Read the model definition and answer for the solid it produces. Units are mm, in the model's axes. Face numbers are marked on the shaded views. A direction names the side the tool comes from. Round coordinates to 2 decimals unless told otherwise and drop trailing zeros. Write each loop counter-clockwise with the first axis right and the second up, starting at its lowest first coordinate (ties: lowest second). Pieces come first, ordered by that corner, then holes. Notation, with made-up numbers: (-9.75, 64) - (19.25, 64) arc R13 ccw to (19.25, 72) - close; hole circle Ø7 at (20.25, 33). An arc over 180 degrees is marked (long way). Answer as CSV lines item,"result". Start each with the question number.
1) Find section B-B on y = 3. Determine the outline of the cut face in (x, z), then the cut area to 3 significant figures.
2) Which of the six approach directions +Z, -Z, +X, -X, +Y, -Y give full straight-line access (tool end or side, diameter ignored) to the marked faces 1, 2 and 3?
3) Find section D-D on x = 53.5. Determine the outline of the cut face in (y, z), then the cut area to 3 significant figures.
4) Each of these flat-tipped pins is pushed along its axis until it touches: pin 1 (6 mm diameter, centred on y = 9.5, z = 21.5, fed in from +X); pin 2 (16 mm diameter, centred on y = 26.5, z = 20, fed in from -X); pin 3 (4 mm diameter, centred on x = 53.5, y = 14.5, fed in from +Z). Where does it stop, or does it pass through?
5) Find section C-C on z = 18. Determine the outline of the cut face in (x, y), then the cut area to 3 significant figures.
6) Find section A-A on x = 2.8. Determine the outline of the cut face in (y, z).
7) Consider line 1 along Y through (x, z) = (53.5, 2.9); line 2 along Y through (x, z) = (2.8, 3.4); line 3 along Y through (x, z) = (48.5, 31.5). Determine where each line is inside the solid, lowest interval first.
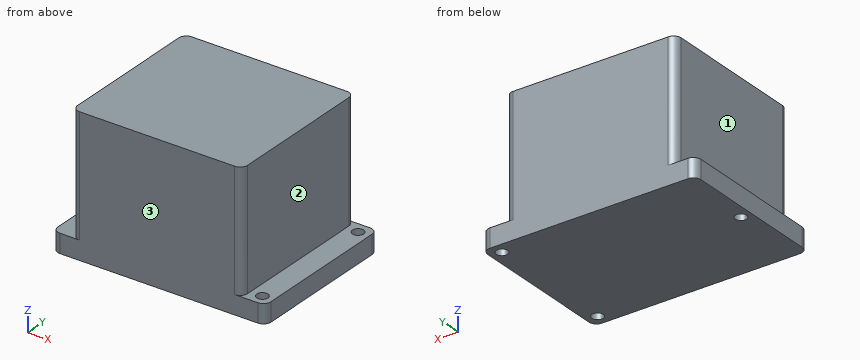
from build123d import *

# Parameters (mm, degrees)
SKETCH_1_W      = 56.5
SKETCH_1_H      = 41
SKETCH_1_R      = 1.5
EXTRUDE_1_DEPTH = 5
FILLET_1_R      = 2
SKETCH_2_W      = 45.103373127
SKETCH_2_H      = 41
EXTRUDE_2_DEPTH = 31.5
FILLET_2_R      = 2


with BuildPart() as part:
    # 草图1 → 凸台-拉伸1 (new body)
    with BuildSketch(Plane.XY):
        with Locations((28.25, 20.5)):
            Rectangle(SKETCH_1_W, SKETCH_1_H)
        with Locations((2.8, 20.5)):
            Circle(SKETCH_1_R, mode=Mode.SUBTRACT)
        with Locations((53.5, 38)):
            Circle(SKETCH_1_R, mode=Mode.SUBTRACT)
        with Locations((53.5, 3)):
            Circle(SKETCH_1_R, mode=Mode.SUBTRACT)
    extrude(amount=EXTRUDE_1_DEPTH)

    # 圆角1
    fillet_1_edges = [part.edges().sort_by_distance(p)[0] for p in [
        (0, 41, 2.5),
        (56.5, 41, 2.5),
        (56.5, 0, 2.5),
        (0, 0, 2.5),
    ]]
    fillet(fillet_1_edges, radius=FILLET_1_R)

    # 草图2 → 凸台-拉伸2 (add)
    with BuildSketch(Plane.XY.offset(5)):
        with Locations((27.783569507, 20.5)):
            Rectangle(SKETCH_2_W, SKETCH_2_H)
    extrude(amount=EXTRUDE_2_DEPTH)

    # 圆角2
    fillet_2_edges = [part.edges().sort_by_distance(p)[0] for p in [
        (50.33525607, 0, 20.75),
        (50.33525607, 41, 20.75),
        (5.231882943, 41, 20.75),
        (5.231882943, 0, 20.75),
    ]]
    fillet(fillet_2_edges, radius=FILLET_2_R)


solid = part.part
Check values:
1,outline,"(0, 0) - (52, 0) - (52, 5) - (50.34, 5) - (50.34, 36.5) - (5.23, 36.5) - (5.23, 5) - (0, 5) - close; (55, 0) - (56.5, 0) - (56.5, 5) - (55, 5) - close"
1,area,"1,690 mm^2"
2,face 1,"+Z, -X, +Y, -Y"
2,face 2,"+Z, +X, +Y, -Y"
2,face 3,"+Z, -Z, +X, -X, -Y"
3,outline,"(0, 0) - (1.5, 0) - (1.5, 5) - (0, 5) - close; (4.5, 0) - (36.5, 0) - (36.5, 5) - (4.5, 5) - close; (39.5, 0) - (41, 0) - (41, 5) - (39.5, 5) - close"
3,area,"175 mm^2"
4,pin 1,"stops at x = 50.34"
4,pin 2,"stops at x = 5.23"
4,pin 3,"stops at z = 5"
5,outline,"(5.23, 2) arc R2 ccw to (7.23, 0) - (48.34, 0) arc R2 ccw to (50.34, 2) - (50.34, 39) arc R2 ccw to (48.34, 41) - (7.23, 41) arc R2 ccw to (5.23, 39) - close"
5,area,"1,850 mm^2"
6,outline,"(0, 0) - (19, 0) - (19, 5) - (0, 5) - close; (22, 0) - (41, 0) - (41, 5) - (22, 5) - close"
7,line 1,"y = 0 to 1.5, 4.5 to 36.5, 39.5 to 41"
7,line 2,"y = 0 to 19, 22 to 41"
7,line 3,"y = 0.01 to 40.99"
